Model file for the job. Use its own axes, mm. Face numbers are marked on the shaded views. Give positions to 0.01 mm unless a question says otherwise; leave off trailing zeros. Write each loop counter-clockwise with the first axis right and the second up, starting at its lowest first coordinate (ties: lowest second). Pieces come first, ordered by that corner, then holes. Notation, with made-up numbers: (30, 64) - (41, 64) arc R19 ccw to (41, 88) - close; hole circle Ø4 at (-36, -4.5). An arc over 180 degrees is marked (long way). One line per item, written item: value. Start each with the question number.
(1) Probe L1, parallel to Y at x = -25, z = -0.55; L2, parallel to Y at x = 25, z = -1.05; L3, parallel to X at y = -2, z = -0.25. List the from-to ranges inside material, lowest first.
(2) Cut at B-B, the plane z = -1.7. List the corners of the cut face in (x, y).
(3) Cut at C-C, the plane y = -6. List the corners of the cut face in (x, z).
(4) Drop a flat-ended pin along its axis: P1, Ø1, axis at y = -4.5, z = 0, coming from the -X side. Give the stop position or say it passes through.
(5) Cut at D-D, the plane x = 28.5. List the corners of the cut face in (y, z).
(6) Mould opens along Z. For the marked faces 1 and 2 say: pulls with the +Z half, pulls with the -Z half, needs draft (parallel to the pull), parting line crosses it, or undercut.
(7) Cut at A-A, the plane y = 0. List the corners of the cut face in (x, z).
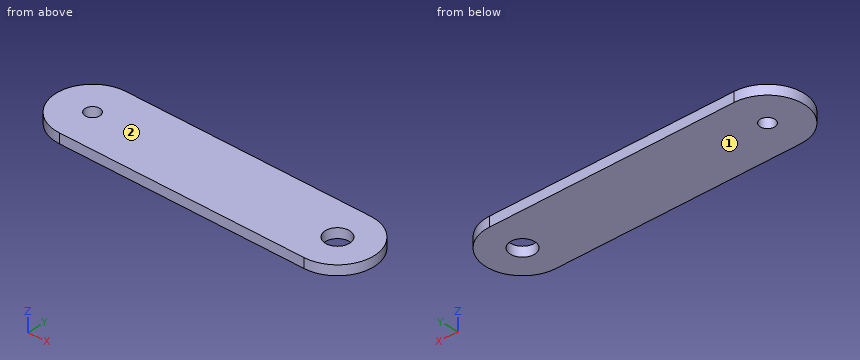
from build123d import *

# Parameters (mm, degrees)
BOSS_EXTRUDE1_DEPTH = 2
CUT_EXTRUDE1_REACH  = 4
SKETCH2_R           = 1.5
SKETCH2_R_2         = 2.5


with BuildPart() as part:
    # Sketch1 → Boss-Extrude1 (new body)
    with BuildSketch(Plane.XY):
        with BuildLine():
            Line((-25, -7.5), (25, -7.5))
            ThreePointArc((25, -7.5), (32.5, 0), (25, 7.5))
            Line((25, 7.5), (-25, 7.5))
            ThreePointArc((-25, 7.5), (-32.5, 0), (-25, -7.5))
        make_face()
    extrude(amount=-BOSS_EXTRUDE1_DEPTH)

    # Sketch2 → Cut-Extrude1 (cut, up to next)
    with BuildSketch(Plane.XY, mode=Mode.PRIVATE) as cut_extrude1_sk1:
        with Locations((-25, 0)):
            Circle(SKETCH2_R)
    cut_extrude1_tool1 = extrude(cut_extrude1_sk1.sketch, amount=-CUT_EXTRUDE1_REACH, mode=Mode.PRIVATE) & part.part
    add(cut_extrude1_tool1.solids().sort_by_distance((-25, 0, 0))[0], mode=Mode.SUBTRACT)
    # Sketch2 → Cut-Extrude1 (cut, up to next)
    with BuildSketch(Plane.XY, mode=Mode.PRIVATE) as cut_extrude1_sk2:
        with Locations((25, 0)):
            Circle(SKETCH2_R_2)
    cut_extrude1_tool2 = extrude(cut_extrude1_sk2.sketch, amount=-CUT_EXTRUDE1_REACH, mode=Mode.PRIVATE) & part.part
    add(cut_extrude1_tool2.solids().sort_by_distance((25, 0, 0))[0], mode=Mode.SUBTRACT)


solid = part.part
Answers follow:
1. L1: y = -7.5 to -1.5, 1.5 to 7.5
1. L2: y = -7.5 to -2.5, 2.5 to 7.5
1. L3: x = -32.23 to 23.5, 26.5 to 32.23
2. outline: (-25, -7.5) - (25, -7.5) arc R7.5 ccw to (25, 7.5) - (-25, 7.5) arc R7.5 ccw to start; hole circle Ø3 at (-25, 0); hole circle Ø5 at (25, 0)
3. outline: (-29.5, -2) - (29.5, -2) - (29.5, 0) - (-29.5, 0) - close
4. P1: stops at x = -31.34
5. outline: (-6.63, -2) - (6.63, -2) - (6.63, 0) - (-6.63, 0) - close
6. face 1: pulls with the -Z half
6. face 2: pulls with the +Z half
7. outline: (-32.5, -2) - (-26.5, -2) - (-26.5, 0) - (-32.5, 0) - close; (-23.5, -2) - (22.5, -2) - (22.5, 0) - (-23.5, 0) - close; (27.5, -2) - (32.5, -2) - (32.5, 0) - (27.5, 0) - close
